from build123d import *

# Parameters (mm, degrees)
BOSS_EXTRU_1_DEPTH      = 3
ENL_V_MAT_EXTRU_1_DEPTH = 10


with BuildPart() as part:
    # Esquisse1 → Boss.-Extru.1 (new body)
    with BuildSketch(Plane.XY):
        Polygon((-129.143746737, -14.701531345), (-206.446773007, -14.701531345), (-222.237416003, -10.173637327), (-228.962816583, -8.245159743), (-323.901077775, 18.972234266), (-327.912092601, 16.748746626), (-350.173506381, -60.88602933), (-347.950273, -64.896848521), (-291.80662177, -80.995781451), (-285.908889082, -97.08692424), (-249.107067355, -113.823629959), (-232.032352152, -131.457901649), (-227.449883961, -131.529994355), (-203.511236428, -108.350948678), (-132.079283315, -108.350948678), (-108.140635782, -131.529994355), (-103.558167591, -131.457901649), (-86.483452388, -113.823629959), (-49.681630661, -97.08692424), (-43.783897973, -80.995781451), (12.359753257, -64.896848521), (14.582986638, -60.88602933), (-7.678427142, 16.748746626), (-11.689441968, 18.972234266), (-106.627703159, -8.245159743), (-113.35310374, -10.173637327), align=None)
        Polygon((-128.0696158, -96.878899722), (-106.057456456, -118.225792128), (-92.935433745, -104.673746846), (-58.425639792, -88.979407851), (-52.188593581, -71.96249534), (1.870889973, -56.461187875), (-14.186085737, -0.463858857), (-50.716621092, -10.938821309), (-52.025991399, -6.372504389), (-70.291259076, -11.609985616), (-70.910965859, -9.448811229), (-90.137733677, -14.960840928), (-89.517720268, -17.123084647), (-107.782987945, -22.360565873), (-107.093845678, -24.763890567), (-125.358331696, -30.001147656), (-111.200088958, -79.377961929), (-127.377713529, -96.161100182), align=None, mode=Mode.SUBTRACT)
        Polygon((-224.390430785, -79.377961929), (-208.212806214, -96.161100182), (-207.491865187, -96.85509979), (-208.236606037, -97.572971364), (-229.533063287, -118.225792128), (-242.655085998, -104.673746846), (-277.164879951, -88.979407851), (-283.401926162, -71.96249534), (-337.461409717, -56.461187875), (-321.404434006, -0.463858857), (-284.873898651, -10.938821309), (-283.564528345, -6.372504389), (-265.299260667, -11.609985616), (-264.679553884, -9.448811229), (-245.452786066, -14.960840928), (-246.072799476, -17.123084647), (-227.807531798, -22.360565873), (-228.496674065, -24.763890567), (-210.232188047, -30.001147656), align=None, mode=Mode.SUBTRACT)
    extrude(amount=BOSS_EXTRU_1_DEPTH)

    # Esquisse2 → Enlèv. mat.-Extru.1 (cut)
    with BuildSketch(Plane.XY.offset(3)):
        with BuildLine():
            Line((-168.795259872, -108.350948678), (-168.795259872, -102.350948678))
            ThreePointArc((-168.795259872, -102.350948678), (-167.795259872, -101.350948678), (-166.795259872, -102.350948678))
            Line((-166.795259872, -102.350948678), (-166.795259872, -108.350948678))
            ThreePointArc((-166.795259872, -108.350948678), (-167.795259872, -109.350948678), (-168.795259872, -108.350948678))
        make_face()
        with BuildLine():
            Line((-164.795259872, -108.350948678), (-164.795259872, -102.350948678))
            ThreePointArc((-164.795259872, -102.350948678), (-163.795259872, -101.350948678), (-162.795259872, -102.350948678))
            Line((-162.795259872, -102.350948678), (-162.795259872, -108.350948678))
            ThreePointArc((-162.795259872, -108.350948678), (-163.795259872, -109.350948678), (-164.795259872, -108.350948678))
        make_face()
        with BuildLine():
            Line((-160.795259872, -108.350948678), (-160.795259872, -102.350948678))
            ThreePointArc((-160.795259872, -102.350948678), (-159.795259872, -101.350948678), (-158.795259872, -102.350948678))
            Line((-158.795259872, -102.350948678), (-158.795259872, -108.350948678))
            ThreePointArc((-158.795259872, -108.350948678), (-159.795259872, -109.350948678), (-160.795259872, -108.350948678))
        make_face()
        with BuildLine():
            Line((-156.795259872, -108.350948678), (-156.795259872, -102.350948678))
            ThreePointArc((-156.795259872, -102.350948678), (-155.795259872, -101.350948678), (-154.795259872, -102.350948678))
            Line((-154.795259872, -102.350948678), (-154.795259872, -108.350948678))
            ThreePointArc((-154.795259872, -108.350948678), (-155.795259872, -109.350948678), (-156.795259872, -108.350948678))
        make_face()
        with BuildLine():
            Line((-152.795259872, -108.350948678), (-152.795259872, -102.350948678))
            ThreePointArc((-152.795259872, -102.350948678), (-151.795259872, -101.350948678), (-150.795259872, -102.350948678))
            Line((-150.795259872, -102.350948678), (-150.795259872, -108.350948678))
            ThreePointArc((-150.795259872, -108.350948678), (-151.795259872, -109.350948678), (-152.795259872, -108.350948678))
        make_face()
        with BuildLine():
            Line((-148.795259872, -108.350948678), (-148.795259872, -102.350948678))
            ThreePointArc((-148.795259872, -102.350948678), (-147.795259872, -101.350948678), (-146.795259872, -102.350948678))
            Line((-146.795259872, -102.350948678), (-146.795259872, -108.350948678))
            ThreePointArc((-146.795259872, -108.350948678), (-147.795259872, -109.350948678), (-148.795259872, -108.350948678))
        make_face()
        with BuildLine():
            Line((-172.795259872, -108.350948678), (-172.795259872, -102.350948678))
            ThreePointArc((-172.795259872, -102.350948678), (-171.795259872, -101.350948678), (-170.795259872, -102.350948678))
            Line((-170.795259872, -102.350948678), (-170.795259872, -108.350948678))
            ThreePointArc((-170.795259872, -108.350948678), (-171.795259872, -109.350948678), (-172.795259872, -108.350948678))
        make_face()
        with BuildLine():
            Line((-176.795259872, -108.350948678), (-176.795259872, -102.350948678))
            ThreePointArc((-176.795259872, -102.350948678), (-175.795259872, -101.350948678), (-174.795259872, -102.350948678))
            Line((-174.795259872, -102.350948678), (-174.795259872, -108.350948678))
            ThreePointArc((-174.795259872, -108.350948678), (-175.795259872, -109.350948678), (-176.795259872, -108.350948678))
        make_face()
        with BuildLine():
            Line((-180.795259872, -108.350948678), (-180.795259872, -102.350948678))
            ThreePointArc((-180.795259872, -102.350948678), (-179.795259872, -101.350948678), (-178.795259872, -102.350948678))
            Line((-178.795259872, -102.350948678), (-178.795259872, -108.350948678))
            ThreePointArc((-178.795259872, -108.350948678), (-179.795259872, -109.350948678), (-180.795259872, -108.350948678))
        make_face()
        with BuildLine():
            Line((-184.795259872, -108.350948678), (-184.795259872, -102.350948678))
            ThreePointArc((-184.795259872, -102.350948678), (-183.795259872, -101.350948678), (-182.795259872, -102.350948678))
            Line((-182.795259872, -102.350948678), (-182.795259872, -108.350948678))
            ThreePointArc((-182.795259872, -108.350948678), (-183.795259872, -109.350948678), (-184.795259872, -108.350948678))
        make_face()
        with BuildLine():
            Line((-188.795259872, -108.350948678), (-188.795259872, -102.350948678))
            ThreePointArc((-188.795259872, -102.350948678), (-187.795259872, -101.350948678), (-186.795259872, -102.350948678))
            Line((-186.795259872, -102.350948678), (-186.795259872, -108.350948678))
            ThreePointArc((-186.795259872, -108.350948678), (-187.795259872, -109.350948678), (-188.795259872, -108.350948678))
        make_face()
    extrude(amount=-ENL_V_MAT_EXTRU_1_DEPTH, mode=Mode.SUBTRACT)


solid = part.part
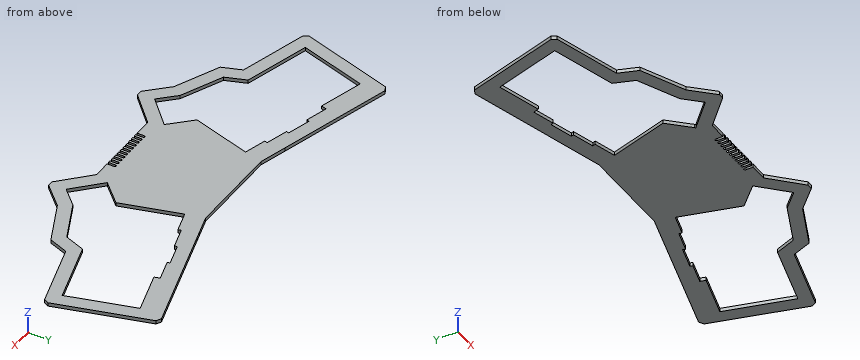
Geometry: final body of the model. Coordinates: model frame, mm. Give positions to 0.01 mm unless a question says otherwise; leave off trailing zeros. Loops run counter-clockwise (first coordinate to the right, second up) from the corner with the lowest first, then second, coordinate; pieces in that order, holes last. Notation, with made-up numbers: M 75.5,39 L 116.5,39 A23 ccw 116.5,53 Z; hole C 89,67 d8. An arc over 180 degrees is marked long. Put each result on its own line as item: value. Start each with the question number.
1) Cut plane A-A (x = -80). Output: boundary loops of the cut face in (y, z).
2) Ray query, line 1 along X through (y, z) = (-56, 2.4); line 2 along X through (y, z) = (-117.5, 1.8); line 3 along X through (y, z) = (-117, 1.85). Return the intervals inside material, ascending.
3) Contact query for flat-ended pins moving along their axis: pin 1 (0.6 mm diameter, centred on x = -166.5, z = 1.5, fed in from -Y); pin 2 (0.9 mm diameter, centred on y = -104, z = 2, fed in from +X); pin 3 (0.9 mm diameter, centred on y = -105.5, z = 1, fed in from -X). Output: stop coordinate, or through.
4) Cut plane B-B (z = 1.1). Give the number of separate pieces and of enclosed holes in the cut face, then the cut area to 3 significant figures.
Verdict:
1. outline: M -110.88,0 L -98.79,0 L -98.79,3 L -110.88,3 Z; M -12.05,0 L -0.61,0 L -0.61,3 L -12.05,3 Z
2. line 1: -348.77 to -337.33, -217.69 to -117.9, 1.74 to 13.18
2. line 2: -245.55 to -230.24, -228.78 to -212.96, -122.63 to -106.81, -105.35 to -90.04
2. line 3: -246.03 to -230.72, -228.27 to -212.44, -123.15 to -107.32, -104.87 to -89.56
3. pin 1: y = -108.35
3. pin 2: x = -63.89
3. pin 3: x = -268.4
4. separate pieces: 1
4. enclosed holes: 2
4. area: 17,500 mm2
